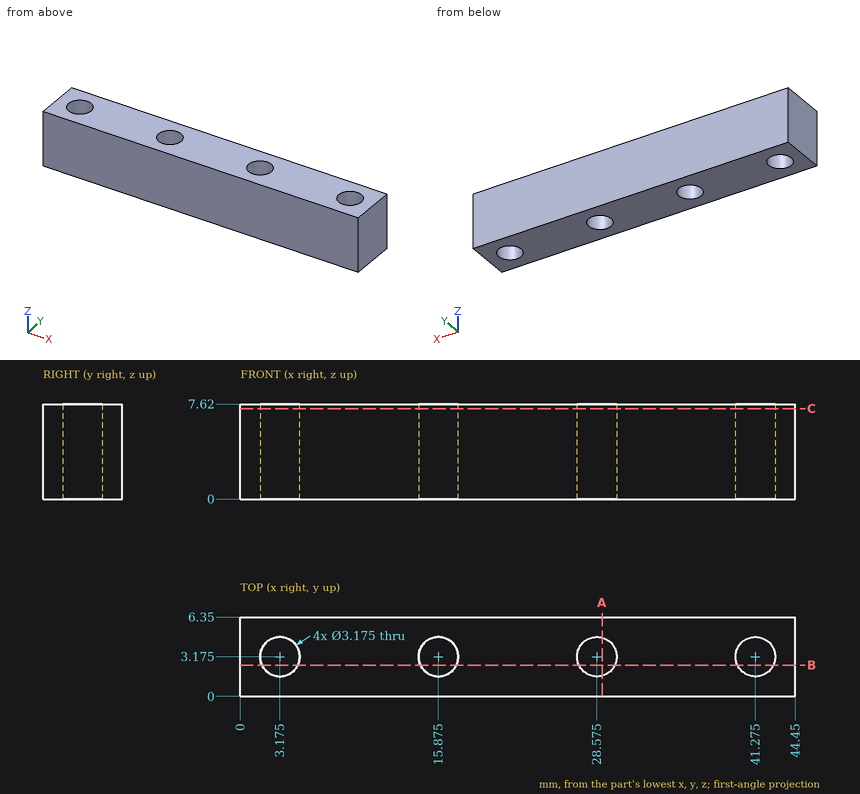
Could you check a few things on this drawing? It's one solid part, dimensions in mm from its lowest x, y, z. Round coordinates to 2 decimals unless told otherwise and drop trailing zeros. Order: outer loops, then holes, each group sorted by start corner. A loop starts at its lowest first (then second) coordinate and runs counter-clockwise, first axis right, second up. Notation, with made-up numbers: M 69,-35 L 94,-35 A8 cw 94,-24 Z; hole C 19.25,40 d7. An arc over 180 degrees is marked long. One line per question, with ' | ' between items. Start each with the question number.
(1) Suppose I cut it at C-C on z = 7.25. Count the separate pieces of the cut face and the enclosed holes in it, then the cut area to 3 significant figures.
(2) Please list where these lines run through material, in increasing order: line 1 along X through (y, z) = (3.75, 7.25); line 2 along X through (y, z) = (2.25, 5.25); line 3 along Y through (x, z) = (27.5, 2).
(3) Suppose I cut it at B-B on y = 2.5. List the corners of the cut face in (x, z) for me.
(4) Suppose I cut it at A-A on x = 29. List the corners of the cut face in (y, z) for me.
Geometry results:
1) separate pieces: 1 | enclosed holes: 4 | area: 251 mm²
2) line 1: 0 to 1.7, 4.65 to 14.4, 17.35 to 27.1, 30.05 to 39.8, 42.75 to 44.45 | line 2: 0 to 1.88, 4.47 to 14.58, 17.17 to 27.28, 29.87 to 39.98, 42.57 to 44.45 | line 3: 0 to 2.01, 4.34 to 6.35
3) outline: M 0,0 L 1.74,0 L 1.74,7.62 L 0,7.62 Z; M 4.61,0 L 14.44,0 L 14.44,7.62 L 4.61,7.62 Z; M 17.31,0 L 27.14,0 L 27.14,7.62 L 17.31,7.62 Z; M 30.01,0 L 39.84,0 L 39.84,7.62 L 30.01,7.62 Z; M 42.71,0 L 44.45,0 L 44.45,7.62 L 42.71,7.62 Z
4) outline: M 0,0 L 1.65,0 L 1.65,7.62 L 0,7.62 Z; M 4.7,0 L 6.35,0 L 6.35,7.62 L 4.7,7.62 Z
